from build123d import *

# Parameters (mm, degrees)
BOSS_EXTRUDE1_DEPTH            = 12.7
CUT_EXTRUDE1_START             = 5
SKETCH2_R                      = 3.3
CUT_EXTRUDE1_DEPTH             = 49.250583245
CUT_EXTRUDE2_DEPTH             = 41.918070929
FILLET1_R                      = 2.1082
FILLET2_R                      = 0.5
SKETCH4_W                      = 7.5
SKETCH4_H                      = 2
SKETCH4_W_2                    = 3
BOSS_EXTRUDE4_DEPTH            = 3
CUT_EXTRUDE3_START             = -5
SKETCH5_R                      = 3.3
CUT_EXTRUDE3_DEPTH             = 50.856761932
CUT_EXTRUDE4_DEPTH             = 44.447671501
CUT_EXTRUDE4_DRAFT             = -1
CUT_EXTRUDE5_REACH             = 45.251
CUT_EXTRUDE5_DIRECTION_2_REACH = 45.251
FILLET3_R                      = 0.5
FILLET4_R                      = 0.5


with BuildPart() as part:
    # Sketch1 → Boss-Extrude1 (new, symmetric)
    with BuildSketch(Plane.XY):
        Polygon((0, 0), (-4.171930009, 4.171930009), (13.788582233, 22.132442251), (34.921024484, 1), (34.921024484, 0), align=None)
    extrude(amount=BOSS_EXTRUDE1_DEPTH, both=True)

    # Sketch2 → Cut-Extrude1 (cut, through all)
    with BuildSketch(Plane(origin=(0, 0, 0), x_dir=(1, 0, 0), z_dir=(0, 1, 0)).offset(CUT_EXTRUDE1_START)):
        with Locations(Location((25.921024484, 0, 0), (0, 0, 270))):
            Circle(SKETCH2_R)
    extrude(amount=-CUT_EXTRUDE1_DEPTH, mode=Mode.SUBTRACT)

    # Sketch3 → Cut-Extrude2 (cut, through all)
    with BuildSketch(Plane.XZ.offset(-5)):
        with BuildLine():
            Line((25.921024484, -6), (35.921024484, -6))
            Line((35.921024484, -6), (35.921024484, 6))
            Line((35.921024484, 6), (25.921024484, 6))
            ThreePointArc((25.921024484, 6), (19.921024484, 0), (25.921024484, -6))
        make_face()
    extrude(amount=-CUT_EXTRUDE2_DEPTH, mode=Mode.SUBTRACT)

    # Fillet1
    fillet1_edges = [part.edges().sort_by_distance(p)[0] for p in [
        (-2.085965005, 2.085965005, -12.7),
        (-2.085965005, 2.085965005, 12.7),
        (24.354803359, 11.566221126, -12.7),
        (24.354803359, 11.566221126, 12.7),
    ]]
    fillet(fillet1_edges, radius=FILLET1_R)

    # Fillet2
    fillet2_edges = [part.edges().sort_by_distance(p)[0] for p in [
        (28.421024484, 5, -6),
        (28.421024484, 5, 6),
        (19.921024484, 5, 0),
    ]]
    fillet(fillet2_edges, radius=FILLET2_R)

    # Sketch4 → Boss-Extrude4 (add, symmetric)
    with BuildSketch(Plane.XY):
        with Locations((3.75, -1)):
            Rectangle(SKETCH4_W, SKETCH4_H)
        with Locations((33.421024484, -1)):
            Rectangle(SKETCH4_W_2, SKETCH4_H)
        Polygon((-4.171930009, 7.000357134), (-2.671930009, 7.000357134), (-2.671930009, 5.671930009), (-4.171930009, 4.171930009), align=None)
        Polygon((10.874368671, 22.046655814), (12.374368671, 22.046655814), (12.374368671, 20.718228689), (10.874368671, 19.218228689), align=None)
    extrude(amount=BOSS_EXTRUDE4_DEPTH, both=True)

    # Sketch5 → Cut-Extrude3 (cut, through all)
    with BuildSketch(Plane(origin=(-4.171930009, 4.171930009, 0), x_dir=(0, 0, 1), z_dir=(-0.7071067811865477, 0.7071067811865475, 0)).offset(CUT_EXTRUDE3_START)):
        with Locations(Location((0, 12.7, 0), (0, 0, 90))):
            Circle(SKETCH5_R)
    extrude(amount=CUT_EXTRUDE3_DEPTH, mode=Mode.SUBTRACT)


with BuildPart() as cut_extrude4_tool:
    # Sketch6 → Cut-Extrude4 (with draft: the straight prism first)
    with BuildSketch(Plane(origin=(-0.636396103, 0.636396103, 0), x_dir=(0, 0, 1), z_dir=(-0.7071067811865476, 0.7071067811865476, 0))):
        with BuildLine():
            Line((-4.25, 12.7), (-4.25, 8.45))
            Line((-4.25, 8.45), (4.25, 8.45))
            Line((4.25, 8.45), (4.25, 12.7))
            ThreePointArc((4.25, 12.7), (0, 16.95), (-4.25, 12.7))
        make_face()
    extrude(amount=-CUT_EXTRUDE4_DEPTH)
    # Cut-Extrude4: the draft: its side faces are tilted about the plane it starts from
    cut_extrude4_sides = [cut_extrude4_tool.faces().sort_by_distance(p)[0] for p in [
        (22.555883071, -7.600574649, -4.25),
        (21.053281161, -9.103176559, 0),
        (22.555883071, -7.600574649, 4.25),
        (27.063688801, -3.092768919, 0),
    ]]
    draft(cut_extrude4_sides, Plane(origin=(-0.636396103, 0.636396103, 0), x_dir=(0, 0, 1), z_dir=(-0.7071067811865476, 0.7071067811865476, 0)), CUT_EXTRUDE4_DRAFT)


with BuildPart() as part_1:
    add(part.part)

    # Cut-Extrude4: cut by cut_extrude4_tool
    add(cut_extrude4_tool.part, mode=Mode.SUBTRACT)

    # Cut-Extrude5: up to this plane
    cut_extrude5_end = Plane(origin=(8.343860018, 9.616652224, 4.25), z_dir=(0.012340714939826952, -0.012340714939826952, 0.9998476951563913))
    # Sketch7 → Cut-Extrude5 (cut, up to the surface)
    with BuildSketch(Plane.XY, mode=Mode.PRIVATE) as cut_extrude5_sk1:
        Polygon((12.185011438, 0), (7.5, 0), (5.338656198, 6.611448404), align=None)
    cut_extrude5_tool1 = split(extrude(cut_extrude5_sk1.sketch, amount=CUT_EXTRUDE5_REACH, mode=Mode.PRIVATE), bisect_by=cut_extrude5_end, keep=Keep.BOTH, mode=Mode.PRIVATE)
    add(cut_extrude5_tool1.solids().sort_by_distance((8.341223, 2.203816, 0))[0], mode=Mode.SUBTRACT)

    # Cut-Extrude5 direction 2: up to this plane
    cut_extrude5_direction_2_end = Plane(origin=(8.343860018, 9.616652224, -4.25), z_dir=(0.012340714939826952, -0.012340714939826952, -0.9998476951563913))
    # Sketch7 → Cut-Extrude5 direction 2 (cut, up to the surface)
    with BuildSketch(Plane.XY, mode=Mode.PRIVATE) as cut_extrude5_direction_2_sk1:
        Polygon((12.185011438, 0), (7.5, 0), (5.338656198, 6.611448404), align=None)
    cut_extrude5_direction_2_tool1 = split(extrude(cut_extrude5_direction_2_sk1.sketch, amount=-CUT_EXTRUDE5_DIRECTION_2_REACH, mode=Mode.PRIVATE), bisect_by=cut_extrude5_direction_2_end, keep=Keep.BOTH, mode=Mode.PRIVATE)
    add(cut_extrude5_direction_2_tool1.solids().sort_by_distance((8.341223, 2.203816, 0))[0], mode=Mode.SUBTRACT)

    # Fillet3
    fillet3_edges = [part_1.edges().sort_by_distance(p)[0] for p in [
        (11.349063838, 12.621856044, 0),
        (6.841258108, 8.114050314, -4.25),
        (6.841258108, 8.114050314, 4.25),
    ]]
    fillet(fillet3_edges, radius=FILLET3_R)

    # Fillet4
    # the kernel refuses this fillet: 0.5 mm, written as the material it adds along each edge
    with BuildSketch(Plane(origin=(7.891440115, -1.197396785, 4.122110611), x_dir=(0.9504313899021286, 0.31083412501895896, -0.007894289860799094), z_dir=(-0.3106893622953352, 0.9503840557787532, 0.015564918183075198))) as fillet4_piece_1_section:
        with BuildLine():
            CenterArc((FILLET4_R * 1.0079266613, FILLET4_R), FILLET4_R, 179.547631009, 90.452368991)
            Line((FILLET4_R * 0.00795782923952, FILLET4_R * 1.0078952463), (0, 0))
            Line((0, 0), (FILLET4_R * 1.0079266613, 0))
        make_face()
    fillet4_piece_1 = extrude(amount=8.905919631, mode=Mode.PRIVATE)
    fillet4_piece_1 = split(fillet4_piece_1, bisect_by=Plane(origin=(6.661619064, 0, 4.078163778), z_dir=(0, 1, 0)), keep=Keep.TOP, mode=Mode.PRIVATE)
    add(fillet4_piece_1)
    with BuildSketch(Plane(origin=(7.891440115, -1.197396785, -4.122110611), x_dir=(-0.004836440394139795, 0.014794442279442568, 0.9998788593234452), z_dir=(-0.3106893622953352, 0.9503840557787532, -0.015564918183075198))) as fillet4_piece_2_section:
        with BuildLine():
            CenterArc((FILLET4_R * 1.0079266613, FILLET4_R), FILLET4_R, 179.547631009, 90.452368991)
            Line((FILLET4_R * 0.00795782923952, FILLET4_R * 1.0078952463), (0, 0))
            Line((0, 0), (FILLET4_R * 1.0079266613, 0))
        make_face()
    fillet4_piece_2 = extrude(amount=8.905919631, mode=Mode.PRIVATE)
    fillet4_piece_2 = split(fillet4_piece_2, bisect_by=Plane(origin=(6.661619064, 0, -4.078163778), z_dir=(0, 1, 0)), keep=Keep.TOP, mode=Mode.PRIVATE)
    add(fillet4_piece_2)


solid = part_1.part
Read the model definition and answer for the solid it produces. Units are mm, in the model's axes. A direction names the side the tool comes from. Round coordinates to 2 decimals unless told otherwise and drop trailing zeros. Write each loop counter-clockwise with the first axis right and the second up, starting at its lowest first coordinate (ties: lowest second). Pieces come first, ordered by that corner, then holes.
Q1. Find section A-A on z = -6.75. Determine the outline of the cut face in (x, y).
Values:
outline: (-4.17, 4.17) - (0, 0) - (34.92, 0) - (34.92, 1) - (13.79, 22.13) - close
Q2. Flat-ended cylindrical pins translate along their axes: P1, Ø10, axis at x = 1, z = 4, coming from the +Y side; P2, Ø1.5, axis at x = 7, y = 18, coming from the -Z side; P3, Ø2.5, axis at y = 20.5, z = 0, coming from the -X side; P4, Ø5.5, axis at x = 23.5, z = -1, coming from the +Y side. Find the tip coordinate at first contact, or state that the pin passes through.
Values:
P1: stops at y = 14.34
P2: passes through
P3: stops at x = 10.87
P4: stops at y = 5
Q3. The mould has two halves that part along X. Classify faces 6 (the face through (17.419, 6.335, 0.09)), 7 (the face through (4.27, 9.03, -0.15)), 8 (the face through (-1.584, 2.435, 12.066)), 9 (the face through (12, 22.047, 0)): released by +X, released by -X, zero draft, split by the parting line, or undercut.
Values:
face 6: undercut
face 7: undercut
face 8: released by -X
face 9: zero draft
Q4. Straight lines are drawn through the part: line 1 (X direction, y = 1.3, z = 0); line 2 (X direction, y = -0.5, z = 1); line 3 (X direction, y = 2.4, z = 0). For each, find the intervals that lie inside material, in ascending order.
Values:
line 1: x = -1.3 to 7.08, 22.28 to 22.62, 29.22 to 34.62
line 2: x = 0 to 7.5, 31.92 to 34.92
line 3: x = -2.4 to 6.72, 21.22 to 22.62, 29.22 to 33.52
Q5. A tool of negligible diameter and unlimited length cuts with its end or side. For faces 1 (the face through (6.6, 3.22, 4.04)), 2 (the face through (-3, 6, 3)), 3 (the face through (7.5, -1, 0)), 4 (the face through (-3, 7, 0)), 5 (the face through (28, 7, -6)), from which of +Z, -Z, +X, -X, +Y, -Y can it reach the whole face along a straight path? Write none if from no direction.
Values:
face 1: none
face 2: +Z, -X, +Y
face 3: +Z, -Z, -Y
face 4: +Z, -Z, -X, +Y
face 5: +X, +Y
